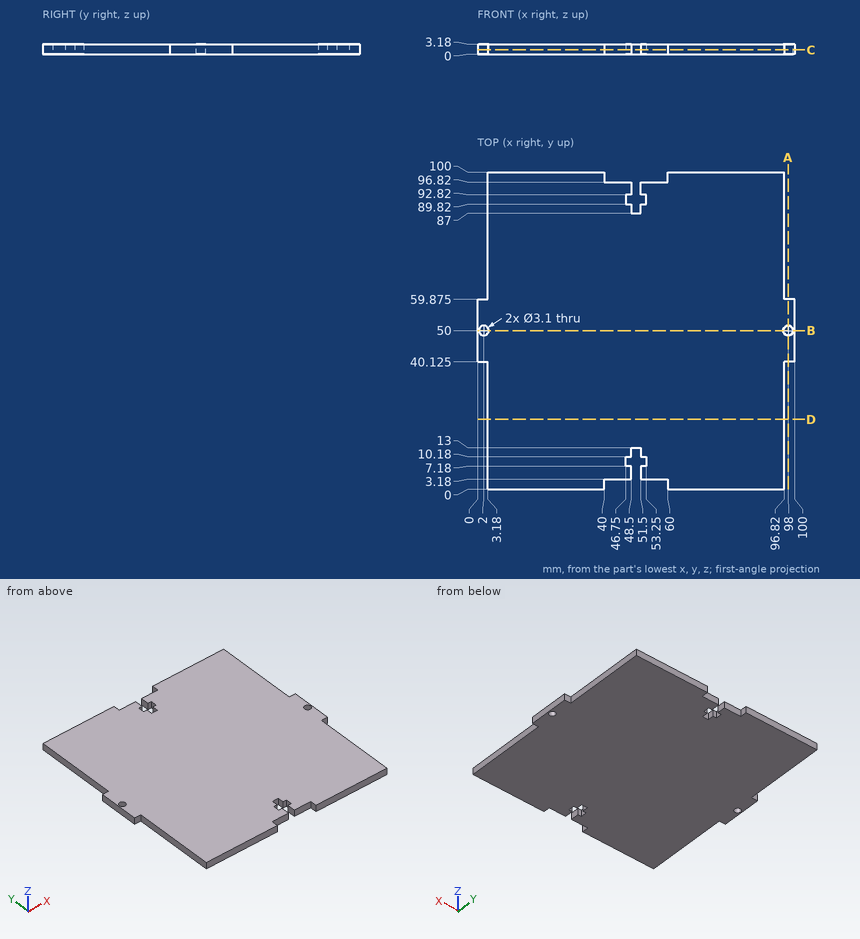
Source: three-view drawing plus pictorial views. Frame: mm from the lowest corner of the part. Round coordinates to 2 decimals unless told otherwise and drop trailing zeros. Loops run counter-clockwise (first coordinate to the right, second up) from the corner with the lowest first, then second, coordinate; pieces in that order, holes last. Notation, with made-up numbers: M 63,85 L 81,85 A35 cw 81,120 Z; hole C 10,-19.5 d5. An arc over 180 degrees is marked long. Put each result on its own line as item: value. Start each with the question number.
(1) Contact query for flat-ended pins moving along their axis: pin 1 Ø1 at (y, z) = (73.5, 1) entering from +X; pin 2 Ø1.5 at (x, z) = (83.5, 1) entering from -Y; pin 3 Ø1.9 at (x, z) = (52, 2) entering from +Y; pin 4 Ø1 at (y, z) = (72, 1.5) entering from -X. Output: stop coordinate, or through.
(2) Material intervals for line 1 along X through (y, z) = (93.5, 2.95); line 2 along X through (y, z) = (72.5, 0.4); line 3 along Y through (x, z) = (98, 1.75) (3 decimals), sorted ascending. Write a range as [from, to].
(3) Section query D-D (y = 22). Return loops of the section in (x, z).
(4) Section query B-B (y = 50). Return loops of the section in (x, z), then the cut area to 3 significant figures.
(5) Section query A-A (x = 98). Return loops of the section in (y, z) (3 decimals), then the cut area to 3 significant figures.
(6) Section query C-C (z = 1.35). State how many separate pieces and enclosed holes the cut face has, then the cut area to 3 significant figures.
Findings below:
1. pin 1: stops at x = 96.82
1. pin 2: stops at y = 0
1. pin 3: stops at y = 96.82
1. pin 4: stops at x = 3.18
2. line 1: x = [3.18, 48.5], [51.5, 96.82]
2. line 2: x = [3.18, 96.82]
2. line 3: y = [40.125, 48.45], [51.55, 59.875]
3. outline: M 3.18,0 L 96.82,0 L 96.82,3.18 L 3.18,3.18 Z
4. outline: M 0,0 L 0.45,0 L 0.45,3.18 L 0,3.18 Z; M 3.55,0 L 96.45,0 L 96.45,3.18 L 3.55,3.18 Z; M 99.55,0 L 100,0 L 100,3.18 L 99.55,3.18 Z
4. area: 298 mm2
5. outline: M 40.125,0 L 48.45,0 L 48.45,3.18 L 40.125,3.18 Z; M 51.55,0 L 59.875,0 L 59.875,3.18 L 51.55,3.18 Z
5. area: 52.9 mm2
6. separate pieces: 1
6. enclosed holes: 2
6. area: 9,270 mm2
